```python
from build123d import *

# Parameters (mm, degrees)
SKETCH2_R           = 4
SKETCH2_W           = 45
SKETCH2_H           = 5
BOSS_EXTRUDE1_DEPTH = 45
SKETCH3_R           = 2
CUT_EXTRUDE1_DEPTH  = 64.765194268


with BuildPart() as part:
    # Sketch2 → Boss-Extrude1 (new body)
    with BuildSketch(Plane(origin=(0, 0, 0), x_dir=(1, 0, 0), z_dir=(0, 1, 0))):
        Circle(SKETCH2_R)
        with Locations((22.5, 0)):
            Rectangle(SKETCH2_W, SKETCH2_H)
    extrude(amount=BOSS_EXTRUDE1_DEPTH)

    # Sketch3 → Cut-Extrude1 (cut, through all)
    with BuildSketch(Plane(origin=(0, 45, 0), x_dir=(1, 0, 0), z_dir=(0, 1, 0))):
        with Locations(Location((0, 0, 0), (0, 0, 270))):
            Circle(SKETCH3_R)
    extrude(amount=-CUT_EXTRUDE1_DEPTH, mode=Mode.SUBTRACT)


solid = part.part
```
Geometry: final body of the model. Coordinates: model frame, mm. A direction names the side the tool comes from. Coordinates: 2 decimals unless noted, no trailing zeros. Order: outer loops, then holes, each group sorted by start corner. A loop starts at its lowest first (then second) coordinate and runs counter-clockwise, first axis right, second up. Notation, with made-up numbers: M 79,81 L 94,81 A24 cw 94,93 Z; hole C 84.25,49 d8. An arc over 180 degrees is marked long. Answer in a Markdown table with one row per item. Add a question column.
Q1. Reachability of faces 1 (the flat face through (20, 0, 0)), 2 (the flat face through (24, 22, 2.5)) from +Z, -Z, +X, -X, +Y, -Y: full face, straight path, thin tool, end or side. Return the list, or none.
Q2. Section query C-C on y = 26. Return the cut outline in (x, z), and give its area (3 significant figures).
Q3. Mould query, pull axis X, two halves, no side actions, for faces 3 (the cylindrical face through (-4, 22, 0)), 4 (the cylindrical face through (-2, 23, 0)), 5 (the flat face through (24, 22, -2.5)). Classes: released by +X, released by -X, zero draft, split by the parting line, or undercut.
Q4. Section query B-B on z = 0. Return the cut outline in (x, y).
Q5. Section query A-A on x = 0. Return the cut outline in (y, z).
Q6. Section query D-D on x = 18.5. Return the cut outline in (y, z).
Q7. Line query: L1, parallel to X at y = 16.5, z = 0; L2, parallel to Z at x = 8, y = 18; L3, parallel to X at y = 15, z = 0.75. Output: solid intervals per line, ascending.
Q8. Contact query for flat-ended pins moving along their axis: P1, Ø1.5, axis at y = 39.5, z = -1, coming from the -X side; P2, Ø10, axis at x = 25, y = 39, coming from the +Z side. Output: stop coordinate, or through.
Completed:
| question | item | result |
|---|---|---|
| 1 | face 1 | +Z, -Z, +X, -X, -Y |
| 1 | face 2 | +Z, +X, +Y, -Y |
| 2 | outline | M 3.12,-2.5 L 45,-2.5 L 45,2.5 L 3.12,2.5 A4 ccw long Z; hole C 0,0 d4 |
| 2 | area | 244 mm2 |
| 3 | face 3 | split by the parting line |
| 3 | face 4 | undercut |
| 3 | face 5 | zero draft |
| 4 | outline | M -4,0 L -2,0 L -2,45 L -4,45 Z; M 2,0 L 45,0 L 45,45 L 2,45 Z |
| 5 | outline | M 0,-4 L 45,-4 L 45,-2 L 0,-2 Z; M 0,2 L 45,2 L 45,4 L 0,4 Z |
| 6 | outline | M 0,-2.5 L 45,-2.5 L 45,2.5 L 0,2.5 Z |
| 7 | L1 | x = -4 to -2, 2 to 45 |
| 7 | L2 | z = -2.5 to 2.5 |
| 7 | L3 | x = -3.93 to -1.85, 1.85 to 45 |
| 8 | P1 | stops at x = -3.99 |
| 8 | P2 | stops at z = 2.5 |
